from build123d import *
from OCP.BRepFilletAPI import BRepFilletAPI_MakeChamfer

# Parameters (mm, degrees)
SKETCH1_W             = 8.255
SKETCH1_H             = 22.225
BOSS_EXTRUDE1_DEPTH   = 6.35
SKETCH2_W             = 6.35
SKETCH2_H             = 4.7625
BOSS_EXTRUDE2_DEPTH   = 6.35
BOSS_EXTRUDE3_START   = -8.255
SKETCH2_4_W           = 6.35
SKETCH2_4_H           = 4.7625
BOSS_EXTRUDE3_DEPTH   = 6.35
SKETCH4_W             = 20.955
SKETCH4_H             = 6.35
BOSS_EXTRUDE4_DEPTH   = 3.135241634
CUT_EXTRUDE3_DEPTH    = 32.199120981
CUT_EXTRUDE4_DEPTH    = 6.35
CUT_EXTRUDE5_START    = -20.955
CUT_EXTRUDE5_DEPTH    = 6.35
F_4_CLEARANCE_HOLE1_D = 3.4544
F_4_CLEARANCE_HOLE2_D = 3.4544
CHAMFER1_SIZE         = 3.175
CHAMFER2_SIZE         = 0.762
CHAMFER2_SIZE2        = 0.737097047
CHAMFER2_SIZE2_2      = 0.789610507


with BuildPart() as part:
    # Sketch1 → Boss-Extrude1 (new body)
    with BuildSketch(Plane.XY):
        with Locations((-57.516108776, -11.1125)):
            Rectangle(SKETCH1_W, SKETCH1_H)
    extrude(amount=BOSS_EXTRUDE1_DEPTH)

    # Sketch2 → Boss-Extrude2 (add)
    with BuildSketch(Plane.ZY.offset(61.643608776)):
        with Locations((3.175, -2.38125)):
            Rectangle(SKETCH2_W, SKETCH2_H)
    extrude(amount=BOSS_EXTRUDE2_DEPTH)

    # Sketch2<4> → Boss-Extrude3 (add)
    with BuildSketch(Plane.ZY.offset(61.643608776).offset(BOSS_EXTRUDE3_START)):
        with Locations((3.175, -2.38125)):
            Rectangle(SKETCH2_4_W, SKETCH2_4_H)
    extrude(amount=-BOSS_EXTRUDE3_DEPTH)

    # Sketch4 → Boss-Extrude4 (add)
    with BuildSketch(Plane(origin=(0, 0, 0), x_dir=(1, 0, 0), z_dir=(0, 1, 0))):
        with Locations((-57.516108776, -3.175)):
            Rectangle(SKETCH4_W, SKETCH4_H)
    extrude(amount=BOSS_EXTRUDE4_DEPTH)

    # Sketch5 → Cut-Extrude3 (cut, through all)
    with BuildSketch(Plane.ZY.offset(67.993608776)):
        Polygon((0, 2.916823594), (6.35, 3.135241634), (0, 3.135241634), align=None)
    extrude(amount=-CUT_EXTRUDE3_DEPTH, mode=Mode.SUBTRACT)

    # Sketch6 → Cut-Extrude4 (cut)
    with BuildSketch(Plane.ZY.offset(67.993608776)):
        Polygon((0, -4.7625), (6.35, -4.54408196), (6.35, -4.7625), align=None)
    extrude(amount=-CUT_EXTRUDE4_DEPTH, mode=Mode.SUBTRACT)

    # Sketch6<2> → Cut-Extrude5 (cut)
    with BuildSketch(Plane.ZY.offset(67.993608776).offset(CUT_EXTRUDE5_START)):
        Polygon((0, -4.7625), (6.35, -4.54408196), (6.35, -4.7625), align=None)
    extrude(amount=CUT_EXTRUDE5_DEPTH, mode=Mode.SUBTRACT)

    # #4 Clearance Hole1 (through all)
    with Locations(Plane(origin=(0, -4.75687204, 0.163619948), x_dir=(-1, 0, 0), z_dir=(0, -0.9994089633576719, 0.03437621212908539))):
        with Locations((50.213608776, -3.013160941), (64.818608776, -3.013160941)):
            Hole(F_4_CLEARANCE_HOLE1_D / 2)

    # #4 Clearance Hole2 (through all)
    with Locations(Plane(origin=(0, 0, 0), x_dir=(-1, 0, 0), z_dir=(0, 0, -1))):
        with Locations((57.516108776, -15.875)):
            Hole(F_4_CLEARANCE_HOLE2_D / 2)

    # Sketch16 → Hole1 (revolve, cut)
    with BuildSketch(Plane(origin=(-57.516108776, -15.875, 0), x_dir=(0, 1, 0), z_dir=(1, 0, 0))):
        Polygon((0, 0), (0, 3.429), (1.9431, 3.429), (2.0701, 0), align=None)
    revolve(axis=Axis((-57.516108776, -15.875, 110), (0, 0, -1)), mode=Mode.SUBTRACT)

    # Chamfer1
    chamfer1_edges = [part.edges().sort_by_distance(p)[0] for p in [
        (-57.516108776, -22.225, 6.35),
    ]]
    chamfer(chamfer1_edges, length=CHAMFER1_SIZE)

    # Chamfer2: one chamfer whose edges measure the first distance from different faces: ONE call of the kernel's chamfer builder (chamfer() names one face for all edges)
    chamfer2_edges_1 = [part.edges().sort_by_distance(p)[0] for p in [
        (-53.388608776, -11.79704098, 6.35),
        (-53.388608776, -22.225, 1.5875),
        (-53.388608776, -20.6375, 4.7625),
        (-61.643608776, -22.225, 1.5875),
        (-61.643608776, -20.6375, 4.7625),
        (-61.643608776, -13.49375, 0),
        (-61.643608776, -11.79704098, 6.35),
        (-47.038608776, -0.704420163, 6.35),
        (-47.038608776, -0.922838203, 0),
        (-67.993608776, -0.922838203, 0),
        (-53.388608776, -13.49375, 0),
        (-57.516108776, -22.225, 0),
        (-67.993608776, -0.704420163, 6.35),
    ]]
    chamfer2_edges_2 = [part.edges().sort_by_distance(p)[0] for p in [
        (-64.818608776, -4.7625, 0),
    ]]
    chamfer2_side_2 = [part.faces().sort_by_distance(p)[0] for p in [
        (-57.516108776, -6.446773357, 0),
    ]]
    chamfer2_edges_3 = [part.edges().sort_by_distance(p)[0] for p in [
        (-50.213608776, -4.7625, 0),
    ]]
    chamfer2_side_3 = [part.faces().sort_by_distance(p)[0] for p in [
        (-50.213608776, -4.759412015, 0.089776027),
    ]]
    chamfer2_edges_4 = [part.edges().sort_by_distance(p)[0] for p in [
        (-57.516108776, 3.135241634, 6.35),
    ]]
    chamfer2_side_4 = [part.faces().sort_by_distance(p)[0] for p in [
        (-57.516108776, -5.076499977, 6.35),
    ]]
    chamfer2_edges_5 = [part.edges().sort_by_distance(p)[0] for p in [
        (-57.516108776, 2.916823594, 0),
    ]]
    chamfer2_side_5 = [part.faces().sort_by_distance(p)[0] for p in [
        (-57.516108776, -6.446773357, 0),
    ]]
    chamfer2_edges_6 = [part.edges().sort_by_distance(p)[0] for p in [
        (-64.818608776, -4.54408196, 6.35),
    ]]
    chamfer2_side_6 = [part.faces().sort_by_distance(p)[0] for p in [
        (-57.516108776, -5.076499977, 6.35),
    ]]
    chamfer2_edges_7 = [part.edges().sort_by_distance(p)[0] for p in [
        (-50.213608776, -4.54408196, 6.35),
    ]]
    chamfer2_side_7 = [part.faces().sort_by_distance(p)[0] for p in [
        (-50.213608776, -4.759412015, 0.089776027),
    ]]
    chamfer2 = BRepFilletAPI_MakeChamfer(part.part.solid().wrapped)
    for e in chamfer2_edges_1:
        chamfer2.Add(CHAMFER2_SIZE, e.wrapped)
    for e in chamfer2_edges_2:
        chamfer2.Add(CHAMFER2_SIZE, CHAMFER2_SIZE2, e.wrapped, chamfer2_side_2[0].wrapped)  # the first distance lies on this face
    for e in chamfer2_edges_3:
        chamfer2.Add(CHAMFER2_SIZE, CHAMFER2_SIZE2, e.wrapped, chamfer2_side_3[0].wrapped)  # the first distance lies on this face
    for e in chamfer2_edges_4:
        chamfer2.Add(CHAMFER2_SIZE, CHAMFER2_SIZE2, e.wrapped, chamfer2_side_4[0].wrapped)  # the first distance lies on this face
    for e in chamfer2_edges_5:
        chamfer2.Add(CHAMFER2_SIZE, CHAMFER2_SIZE2_2, e.wrapped, chamfer2_side_5[0].wrapped)  # the first distance lies on this face
    for e in chamfer2_edges_6:
        chamfer2.Add(CHAMFER2_SIZE, CHAMFER2_SIZE2_2, e.wrapped, chamfer2_side_6[0].wrapped)  # the first distance lies on this face
    for e in chamfer2_edges_7:
        chamfer2.Add(CHAMFER2_SIZE, CHAMFER2_SIZE2_2, e.wrapped, chamfer2_side_7[0].wrapped)  # the first distance lies on this face
    add(Compound.cast(chamfer2.Shape()), mode=Mode.REPLACE)


solid = part.part
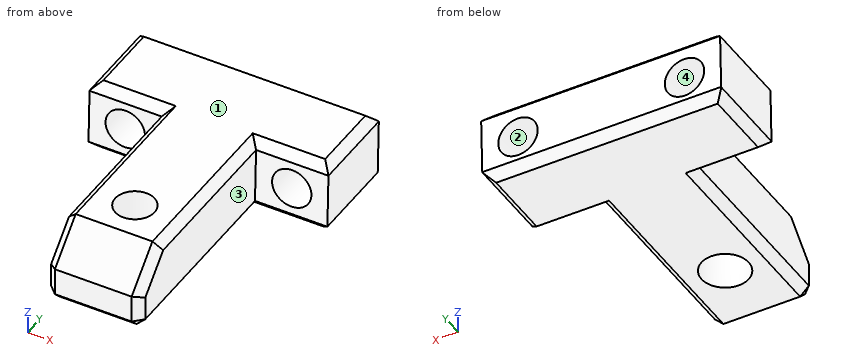
Work out the finished part from the listing and answer in its coordinate system (mm). Face numbers are marked on the shaded views. Give positions to 0.01 mm unless a question says otherwise; leave off trailing zeros. Loops run counter-clockwise (first coordinate to the right, second up) from the corner with the lowest first, then second, coordinate; pieces in that order, holes last. Notation, with made-up numbers: M 47.5,36.25 L 79.5,36.25 A16 ccw 79.5,45.25 Z; hole C 29,-17 d5. An arc over 180 degrees is marked long. Use CSV: the item, a comma, the result in double quotes.
1) Determine the mould class of the marked faces 1, 2, 3 and 4 for opening direction Z: released by +Z, released by -Z, zero draft, split by the parting line, or undercut.
Answer:
face 1,"released by +Z"
face 2,"undercut"
face 3,"zero draft"
face 4,"undercut"
2) Consider L1, parallel to X at y = -4, z = 3.5; L2, parallel to X at y = -18.25, z = 3.75; L3, parallel to Y at x = -57.75, z = 1.5 (3 decimals). Determine where each line is inside the solid, lowest interval first.
Answer:
L1,"-67.99 to -66.51, -63.13 to -51.91, -48.52 to -47.04"
L2,"-61.64 to -53.39"
L3,"-22.225 to -17.876, -13.874 to 2.968"
3) Find section B-B on y = -12. Write down the section's boundary in (x, z).
Answer:
outline,"M -61.64,0.76 L -60.88,0 L -54.15,0 L -53.39,0.76 L -53.39,5.59 L -54.15,6.35 L -60.88,6.35 L -61.64,5.59 Z"
4) Find section C-C on z = 4.5. Give the number of separate pieces and of enclosed holes in the cut face, plus the area to 3 significant figures.
Answer:
separate pieces,"3"
enclosed holes,"1"
area,"257 mm^2"
5) Given P1, Ø1.5, axis at y = -11.5, z = 0.5, coming from the -X side; P2, Ø3, axis at x = -51.5, y = -8, coming from the +Z side; P3, Ø10, axis at x = -50.5, y = -18.5, coming from the +Z side, each flat-ended and moving along its own axis, determine where each tip first touches the part or whether it passes through.
Answer:
P1,"x = -61.64"
P2,"through"
P3,"z = 6.35"
6) Find section A-A on x = -52.75. Write down the section's boundary in (y, z), plus the area to 3 significant figures.
Answer:
outline,"M -4.74,0.76 L -4.03,0 L 2.15,0 L 2.94,0.79 L 3.11,5.61 L 2.37,6.35 L -3.75,6.35 L -4.57,5.59 Z"
area,"47.6 mm^2"
